Source: CAD feature listing. Evaluate the final solid. Frame: model axes, mm. A direction names the side the tool comes from. Give positions to 0.01 mm unless a question says otherwise; leave off trailing zeros. Write each loop counter-clockwise with the first axis right and the second up, starting at its lowest first coordinate (ties: lowest second). Pieces come first, ordered by that corner, then holes. Notation, with made-up numbers: M 17,-13 L 45,-13 A23 ccw 45,26 Z; hole C 35,64 d11. An arc over 180 degrees is marked long. Return JSON: item names as keys, results as strings.
```python
from build123d import *

# Parameters (mm, degrees)
F0_R          = 40.64
F0_R_2        = 34.29
F1_DEPTH      = 120.65
F2_DEPTH      = 6.35
F3_R          = 4.7625
F4_DEPTH      = 50.8
F4_DEPTH_BACK = 50.8
F2_FACE_R     = 34.29
F5_DEPTH      = 114.301


with BuildPart() as f1:
    # F0 (on Top) → F1 (new body)
    with BuildSketch(Plane.XY):
        Circle(F0_R)
        Circle(F0_R_2, mode=Mode.SUBTRACT)
    extrude(amount=F1_DEPTH)

    # F0 (on Top) → F2 (join)
    with BuildSketch(Plane.XY):
        Circle(F0_R_2)
    extrude(amount=F2_DEPTH)

    # F3 (on Front) → F4 (join, two sides)
    with BuildSketch(Plane.XZ) as f4_sk:
        with Locations((0, 107.95)):
            Circle(F3_R)
    extrude(amount=F4_DEPTH)
    extrude(f4_sk.sketch, amount=-F4_DEPTH_BACK)

    # F2_face (on face) → F5 (cut, through all)
    with BuildSketch(Plane.XY.offset(6.35)):
        Circle(F2_FACE_R)
    extrude(amount=F5_DEPTH, mode=Mode.SUBTRACT)


solid = f1.part
```
1) Cut plane A-A, the plane z = 107.95. Return the cut outline in (x, y).
Numbers:
{"outline": "M -4.76,-50.8 L 4.76,-50.8 L 4.76,-40.36 A40.64 ccw 4.76,40.36 L 4.76,50.8 L -4.76,50.8 L -4.76,40.36 A40.64 ccw -4.76,-40.36 Z; hole C 0,0 d68.58"}
2) Draft query along X for faces 3 (the face through (-18, -30, 120.65)), 4 (the face through (0, 0, 6.35)), 5 (the face through (-1.03, 45.51, 103.3)). Return one class per face: released by +X, released by -X, zero draft, split by the parting line, or undercut.
Numbers:
{"face 3": "zero draft", "face 4": "undercut", "face 5": "split by the parting line"}
3) Contact query for flat-ended pins moving along their axis: pin 1 Ø3 at (y, z) = (5, 90) entering from +X; pin 2 Ø12 at (y, z) = (33, 71) entering from -X; pin 3 Ø1.5 at (x, z) = (8.5, 35) entering from -Y. Output: stop coordinate, or through.
Numbers:
{"pin 1": "stops at x = 40.49", "pin 2": "stops at x = -30.37", "pin 3": "stops at y = -39.89"}
4) Cut plane C-C, the plane x = 0. Return the cut outline in (y, z).
Numbers:
{"outline": "M -50.8,103.19 L -40.64,103.19 L -40.64,0 L 40.64,0 L 40.64,103.19 L 50.8,103.19 L 50.8,112.71 L 40.64,112.71 L 40.64,120.65 L 34.29,120.65 L 34.29,6.35 L -34.29,6.35 L -34.29,120.65 L -40.64,120.65 L -40.64,112.71 L -50.8,112.71 Z"}
5) Line query: line 1 (Y direction, x = 0, z = 93.5); line 2 (X direction, y = -1, z = 14.5); line 3 (Z direction, x = 10.5, y = 18). Output: solid intervals per line, ascending. Write a range as [from, to].
Numbers:
{"line 1": "y = [-40.64, -34.29], [34.29, 40.64]", "line 2": "x = [-40.63, -34.28], [34.28, 40.63]", "line 3": "z = [0, 6.35]"}
6) Cut plane D-D, the plane y = -29. Return the cut outline in (x, z).
Numbers:
{"outline": "M -28.47,0 L 28.47,0 L 28.47,120.65 L 18.3,120.65 L 18.3,6.35 L -18.3,6.35 L -18.3,120.65 L -28.47,120.65 Z"}
7) Set-up query: faces 1 (the face through (-1.03, -45.51, 103.3)), 2 (the face through (0, -50.8, 108)). Return all of +Z, -Z, +X, -X, +Y, -Y with unobstructed straight access to the full face (end or side cutting, diameter ignored); none if empty.
Numbers:
{"face 1": "-Y", "face 2": "+Z, -Z, +X, -X, -Y"}
8) Cut plane B-B, the plane y = 0. Return the cut outline in (x, z), then the cut area to 3 significant figures.
Numbers:
{"outline": "M -40.64,0 L 40.64,0 L 40.64,120.65 L 34.29,120.65 L 34.29,6.35 L -34.29,6.35 L -34.29,120.65 L -40.64,120.65 Z", "area": "1,970 mm²"}
